Can you work these out from the model? Positions are in its coordinate system, mm. Face numbers are marked on the shaded views. A direction names the side the tool comes from. Coordinates: 2 decimals unless noted, no trailing zeros. Order: outer loops, then holes, each group sorted by start corner. A loop starts at its lowest first (then second) coordinate and runs counter-clockwise, first axis right, second up. Notation, with made-up numbers: (-7.5, 69.5) - (30.5, 69.5) arc R23 ccw to (30.5, 91.5) - close; hole circle Ø3 at (-18, -37.75). An arc over 180 degrees is marked (long way). Use a Markdown table: item, result. Add a question column.
(1) I want a section at D-D (z = 39.5). List the corners of the cut face in (x, y) for me, and give its area (3 significant figures).
(2) On a 3-axis mill with a long thin cutter (end or side, diameter ignored), from which of +Z, -Z, +X, -X, +Y, -Y can I reach the whole of each face in a straight line? I mean the marked faces 4 and 5. Say none if no direction works.
(3) If I drill on L1, parallel to X at y = 166.5, z = 46; L2, parallel to Y at x = 61.5, z = 46.75; L3, parallel to X at y = 169, z = 43, over which ranges is the centre line in solid material (lowest first)? Write a range as [from, to].
(4) We'd pull the mould along Y, two halves only. Please class the marked faces 1, 2 and 3: pulls with the +Y half, pulls with the -Y half, needs draft (parallel to the pull), parting line crosses it, or undercut.
(5) I want a section at B-B (y = 166.5). List the corners of the cut face in (x, z) for me.
(6) I want a section at C-C (z = 47.25). List the corners of the cut face in (x, y) for me, and give its area (3 significant figures).
(7) I want a section at A-A (x = 69.5). List the corners of the cut face in (y, z) for me.
```python
from build123d import *

# Parameters (mm, degrees)
SKETCH_1_W      = 40
SKETCH_1_H      = 10
SKETCH_1_R      = 2.3
EXTRUDE_1_DEPTH = 10
SKETCH_2_W      = 12
SKETCH_2_H      = 10
EXTRUDE_3_DEPTH = 100
SKETCH_3_W      = 40
SKETCH_3_H      = 10
SKETCH_3_R      = 2.329290182
EXTRUDE_4_DEPTH = 10
CHAMFER_1_SIZE  = 5


with BuildPart() as part:
    # Эскиз1 → Бобышка-Вытянуть1 (new body)
    with BuildSketch(Plane(origin=(0, 116.195974268, 0), x_dir=(1, 0, 0), z_dir=(0, 1, 0))):
        with Locations((64.808980694, -43.273129836)):
            Rectangle(SKETCH_1_W, SKETCH_1_H)
        with Locations(Location((64.808980694, -43.273129836, 0), (0, 0, 180))):
            Circle(SKETCH_1_R, mode=Mode.SUBTRACT)
    extrude(amount=EXTRUDE_1_DEPTH)

    # Эскиз2 → Бобышка-Вытянуть3 (add)
    with BuildSketch(Plane(origin=(0, 126.195974268, 0), x_dir=(1, 0, 0), z_dir=(0, 1, 0))):
        with Locations((50.808980694, -43.273129836)):
            Rectangle(SKETCH_2_W, SKETCH_2_H)
        with Locations((78.808980694, -43.273129836)):
            Rectangle(SKETCH_2_W, SKETCH_2_H)
    extrude(amount=EXTRUDE_3_DEPTH)

    # Эскиз3 → Бобышка-Вытянуть4 (add)
    with BuildSketch(Plane(origin=(0, 226.195974268, 0), x_dir=(1, 0, 0), z_dir=(0, 1, 0))):
        with Locations((64.808980694, -43.273129836)):
            Rectangle(SKETCH_3_W, SKETCH_3_H)
        with Locations(Location((64.808980694, -43.273129836, 0), (0, 0, 180))):
            Circle(SKETCH_3_R, mode=Mode.SUBTRACT)
    extrude(amount=EXTRUDE_4_DEPTH)

    # Фаска1
    chamfer_1_edges = [part.edges().sort_by_distance(p)[0] for p in [
        (44.808980694, 176.195974268, 38.273129836),
        (84.808980694, 176.195974268, 38.273129836),
    ]]
    chamfer(chamfer_1_edges, length=CHAMFER_1_SIZE)


solid = part.part
```
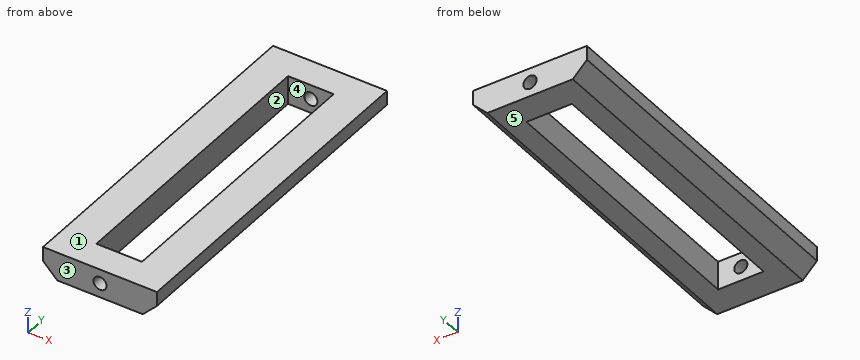
Answers follow:
| question | item | result |
|---|---|---|
| 1 | outline | (48.58, 116.2) - (81.04, 116.2) - (81.04, 236.2) - (48.58, 236.2) - close; hole (56.81, 126.2) - (72.81, 126.2) - (72.81, 226.2) - (56.81, 226.2) - close |
| 1 | area | 2,290 mm² |
| 2 | face 4 | +Z, -Z |
| 2 | face 5 | -Z, +X, -X, +Y, -Y |
| 3 | L1 | x = [44.81, 56.81], [72.81, 84.81] |
| 3 | L2 | y = [116.2, 126.2], [226.2, 236.2] |
| 3 | L3 | x = [45.08, 56.81], [72.81, 84.54] |
| 4 | face 1 | needs draft |
| 4 | face 2 | undercut |
| 4 | face 3 | pulls with the -Y half |
| 5 | outline | (44.81, 43.27) - (49.81, 38.27) - (56.81, 38.27) - (56.81, 48.27) - (44.81, 48.27) - close; (72.81, 38.27) - (79.81, 38.27) - (84.81, 43.27) - (84.81, 48.27) - (72.81, 48.27) - close |
| 6 | outline | (44.81, 116.2) - (84.81, 116.2) - (84.81, 236.2) - (44.81, 236.2) - close; hole (56.81, 126.2) - (72.81, 126.2) - (72.81, 226.2) - (56.81, 226.2) - close |
| 6 | area | 3,200 mm² |
| 7 | outline | (116.2, 38.27) - (126.2, 38.27) - (126.2, 48.27) - (116.2, 48.27) - close; (226.2, 38.27) - (236.2, 38.27) - (236.2, 48.27) - (226.2, 48.27) - close |
